Here's the drawing with two shaded views (mm, measured from the low corner). I have some questions. A direction names the side the tool comes from. Round coordinates to 2 decimals unless told otherwise and drop trailing zeros. Write each loop counter-clockwise with the first axis right and the second up, starting at its lowest first coordinate (ties: lowest second). Pieces come first, ordered by that corner, then holes. Notation, with made-up numbers: (50, 69.25) -> (54, 69.25) arc R13 cw to (54, 83.25) -> close; hole circle Ø10 at (-40, 65). An arc over 180 degrees is marked (long way). Use CSV: the item, a comma, the result in double quotes.
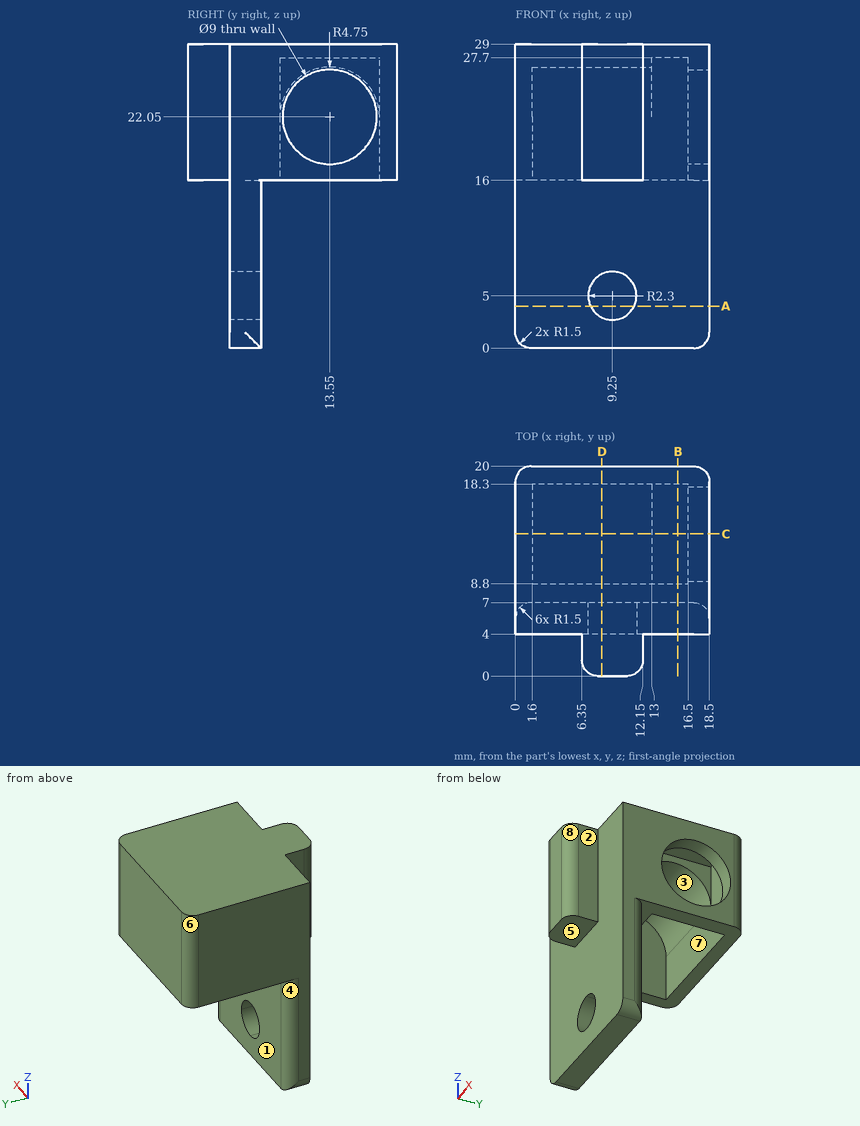
Q1. Suppose I cut it at B-B (x = 15.5). Write out the boundary of the cut face in (y, z), and give its area (3 significant figures).
Resolved:
outline,"(4, 0) -> (7, 0) -> (7, 16) -> (8.8, 16) -> (8.8, 27.7) -> (18.3, 27.7) -> (18.3, 16) -> (20, 16) -> (20, 29) -> (4, 29) -> close"
area,"145 mm^2"
Q2. On a 3-axis mill with a long thin cutter (end or side, diameter ignored), from which of +Z, -Z, +X, -X, +Y, -Y can I reach the whole of each face in a straight line? I mean the marked faces 1, 2, 3, 4 and 5. Say none if no direction works.
Resolved:
face 1,"-Z, +X, -X, +Y"
face 2,"+Z, -Z, +X, -Y"
face 3,"-Z"
face 4,"-Z, -X, +Y"
face 5,"-Z, +X, -X, -Y"
Q3. Suppose I cut it at A-A (z = 4). Write out the boundary of the cut face in (x, y).
Resolved:
outline,"(0, 4) -> (7.18, 4) -> (7.18, 7) -> (1.5, 7) arc R1.5 ccw to (0, 5.5) -> close; (11.32, 4) -> (18.5, 4) -> (18.5, 5.5) arc R1.5 ccw to (17, 7) -> (11.32, 7) -> close"
Q4. If we mould it in two halves opening along X, with no side actions, what happens to the marked faces 6, 7 and 8? For each: released by +X, released by -X, zero draft, split by the parting line, or undercut.
Resolved:
face 6,"released by -X"
face 7,"undercut"
face 8,"released by +X"
Q5. Suppose I cut it at C-C (y = 13.55). Write out the boundary of the cut face in (x, z).
Resolved:
outline,"(0, 16) -> (1.6, 16) -> (1.6, 26.8) -> (13, 26.8) -> (13, 27.7) -> (16.5, 27.7) -> (16.5, 26.55) -> (18.5, 26.55) -> (18.5, 29) -> (0, 29) -> close; (16.5, 16) -> (18.5, 16) -> (18.5, 17.55) -> (16.5, 17.55) -> close"
Q6. Suppose I cut it at D-D (x = 8.25). Write out the boundary of the cut face in (y, z), and give its area (3 significant figures).
Resolved:
outline,"(0, 16) -> (4, 16) -> (4, 7.07) -> (7, 7.07) -> (7, 16) -> (8.8, 16) -> (8.8, 22.05) arc R4.75 cw to (18.3, 22.05) -> (18.3, 16) -> (20, 16) -> (20, 29) -> (0, 29) -> close; (4, 0) -> (7, 0) -> (7, 2.93) -> (4, 2.93) -> close"
area,"203 mm^2"
Q7. Will these pins go through, and if not, where does the flat tip stop? P1, Ø5.5, axis at x = 11.5, z = 20.5, coming from the -Y side; P2, Ø0.8, axis at y = 2.5, z = 19.5, coming from the +X side; P3, Ø4.5, axis at x = 10.5, y = 1.5, coming from the -Z side; P4, Ø3, axis at y = 13, z = 23.5, coming from the +X side.
Resolved:
P1,"stops at y = 0"
P2,"stops at x = 12.15"
P3,"stops at z = 16"
P4,"stops at x = 1.6"
Q8. Please list where these lines run through material, in increasing order: probe 1 along Y at (x, z) = (17.1, 22.05); probe 2 along X at (y, z) = (16.5, 27.5); probe 3 along Z at (x, y) = (15.5, 18).
Resolved:
probe 1,"y = 4 to 9.05, 18.05 to 20"
probe 2,"x = 0 to 13, 16.5 to 18.5"
probe 3,"z = 27.7 to 29"
